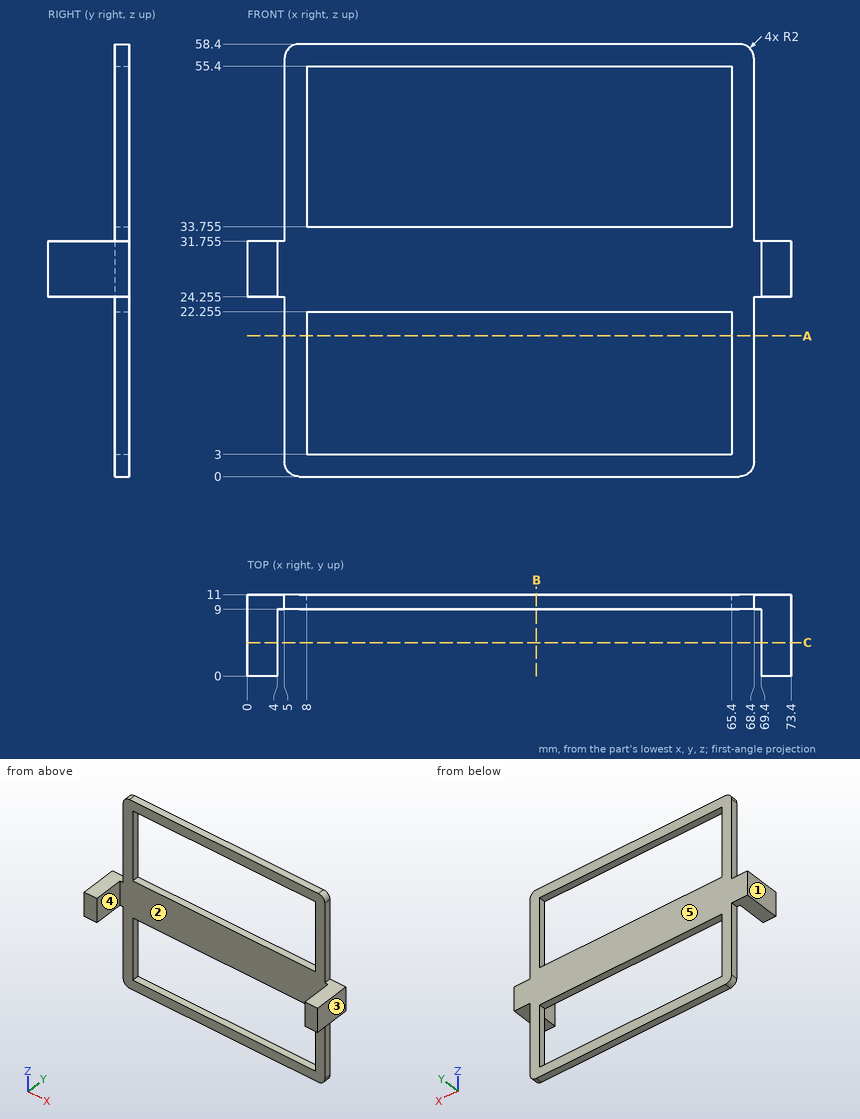
Verification items for this drawing (mm, ordinates from the low corner). A direction names the side the tool comes from. Coordinates: 2 decimals unless noted, no trailing zeros. Order: outer loops, then holes, each group sorted by start corner. A loop starts at its lowest first (then second) coordinate and runs counter-clockwise, first axis right, second up. Notation, with made-up numbers: M -21.5,27 L 11.5,27 A34 cw 11.5,65 Z; hole C 32.25,62 d10. An arc over 180 degrees is marked long. Answer as a JSON object with one key per item and string values.
Q1. Release check for a two-part mould opening along X. For the marked faces 3, 4 and 5 record: released by +X, released by -X, zero draft, split by the parting line, or undercut.
Results are:
{"face 3": "released by +X", "face 4": "undercut", "face 5": "zero draft"}
Q2. Cross-section at A-A on z = 19. Record the cut outline in (x, y).
Results are:
{"outline": "M 5,9 L 8,9 L 8,11 L 5,11 Z; M 65.4,9 L 68.4,9 L 68.4,11 L 65.4,11 Z"}
Q3. Cross-section at B-B on x = 39. Record the cut outline in (y, z) (3 decimals), and give its area (3 significant figures).
Results are:
{"outline": "M 9,0 L 11,0 L 11,3 L 9,3 Z; M 9,22.255 L 11,22.255 L 11,33.755 L 9,33.755 Z; M 9,55.4 L 11,55.4 L 11,58.4 L 9,58.4 Z", "area": "35.0 mm²"}
Q4. Tool access check on the marked faces 1 and 2. Record the directions out of +Z, -Z, +X, -X, +Y, -Y that give a thin tool (end or side, any length) a straight path to the whole face; none if there is none.
Results are:
{"face 1": "+Z, -Z, -X, +Y, -Y", "face 2": "+Z, -Z, -Y"}
Q5. Scan lines: line 1 (Z direction, x = 24.5, y = 9.75) (3 decimals); line 2 (X direction, y = 9.25, z = 44.5); line 3 (X direction, y = 5.75, z = 26). Record each from-to range of solid material in increasing order.
Results are:
{"line 1": "z = 0 to 3, 22.255 to 33.755, 55.4 to 58.4", "line 2": "x = 5 to 8, 65.4 to 68.4", "line 3": "x = 0 to 4, 69.4 to 73.4"}
Q6. Cross-section at C-C on y = 4.5. Record the cut outline in (x, z) (3 decimals).
Results are:
{"outline": "M 0,24.255 L 4,24.255 L 4,31.755 L 0,31.755 Z; M 69.4,24.255 L 73.4,24.255 L 73.4,31.755 L 69.4,31.755 Z"}
Q7. Depth check by flat-ended pin: pin 1 Ø1.6 at (y, z) = (10.5, 8.5) entering from -X; pin 2 Ø17.5 at (x, z) = (33.5, 35.5) entering from -Y; pin 3 Ø1.5 at (x, y) = (71, 7.5) entering from +Z (3 decimals); pin 4 Ø12 at (x, z) = (48.5, 14) entering from -Y. Enter the tip coordinate at first touch or a pass-through.
Results are:
{"pin 1": "stops at x = 5", "pin 2": "stops at y = 9", "pin 3": "stops at z = 31.755", "pin 4": "passes through"}
